```python
from build123d import *

# Parameters (mm, degrees)
CROQUIS3_R            = 2.25
CROQUIS3_R_2          = 1.25
CORTAR_EXTRUIR1_DEPTH = 2.5
CORTAR_EXTRUIR2_DEPTH = 8


with BuildPart() as part:
    # Croquis2 → Revolución1 (revolve)
    with BuildSketch(Plane.XY):
        Polygon((0, 0), (1, 0), (1, 2.05), (6.75, 2.05), (6.75, 6.05), (1, 6.05), (1, 8.1), (12.4, 8.1), (12.4, 61.6), (3.5, 61.6), (3.5, 64.2), (2, 64.2), (2, 73.7), (0, 73.7), align=None)
    revolve(axis=Axis((0, 73.7, 0), (0, -1, 0)))

    # Croquis3 → Cortar-Extruir1 (cut)
    with BuildSketch(Plane(origin=(0, 61.6, 0), x_dir=(1, 0, 0), z_dir=(0, 1, 0))):
        with Locations((8.75, 0)):
            Circle(CROQUIS3_R)
        with Locations((-8.75, 0)):
            Circle(CROQUIS3_R)
        with Locations((0, 8.5)):
            Circle(CROQUIS3_R_2)
        with Locations((0, -8.5)):
            Circle(CROQUIS3_R_2)
    extrude(amount=-CORTAR_EXTRUIR1_DEPTH, mode=Mode.SUBTRACT)

    # Croquis4 → Cortar-Extruir2 (cut)
    with BuildSketch(Plane(origin=(0, 73.7, 0), x_dir=(1, 0, 0), z_dir=(0, 1, 0))):
        Polygon((1.5, 50.388324137), (1.5, 1.322875656), (1.5, -1.322875656), (1.5, -50.388324137), (99.630896962, -50.388324137), (99.630896962, 50.388324137), align=None)
    extrude(amount=-CORTAR_EXTRUIR2_DEPTH, mode=Mode.SUBTRACT)


solid = part.part
```
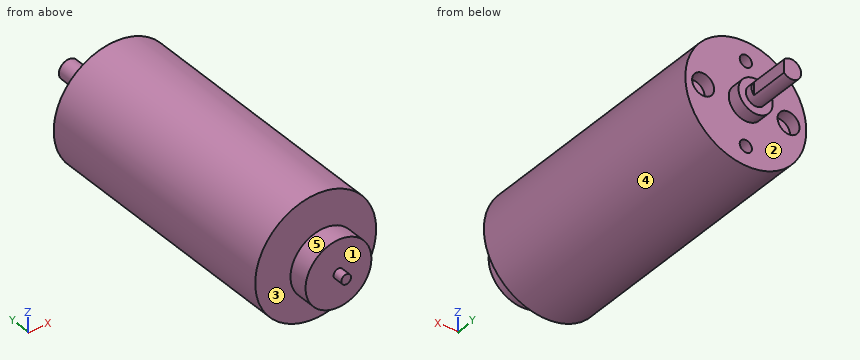
CAD build for the part. Positions are in the model's coordinates, mm. Face numbers are marked on the shaded views. A direction names the side the tool comes from. Round coordinates to 2 decimals unless told otherwise and drop trailing zeros. Order: outer loops, then holes, each group sorted by start corner. A loop starts at its lowest first (then second) coordinate and runs counter-clockwise, first axis right, second up.
Q1. Slice it at D-D (y = 39.5). Write the cut outline in (x, z), and give its area (3 significant figures).
Q2. Slice it at B-B (x = -10). Write the cut outline in (y, z), and give its area (3 significant figures).
Q3. Drop flat-ended pins along their axis: pin 1 (8 mm diameter, centred on y = 15, z = 6, fed in from +X); pin 2 (4 mm diameter, centred on x = 8.75, z = 0, fed in from +Y); pin 3 (2 mm diameter, centred on y = 48.5, z = -6, fed in from -X). Give the stop position or say it passes through.
Q4. Wall check: L1, parallel to Z at x = 0, y = 60.75; L2, parallel to Y at x = -2, z = -4.5; L3, parallel to Y at x = 8.5, z = 0.75. Give the ranges that are in metal, low to high.
Q5. Two-plate mould, pull along Y, no slides. Class the marked faces 1, 2 and 3: pulls with the +Y half, pulls with the -Y half, needs draft (parallel to the pull), parting line crosses it, or undercut.
Q6. Slice it at C-C (x = 5.75). Write the cut outline in (y, z).
Q7. Which spindle directions (+Z, -Z, +X, -X, +Y, -Y) get a long thin tool onto all of the face, cutting with end or side? Do the marked faces 4 and 5. Say none if no direction does.
Results below:
1. outline: circle Ø24.8 at (0, 0)
1. area: 483 mm2
2. outline: (8.1, -7.33) - (61.6, -7.33) - (61.6, -1.87) - (59.1, -1.87) - (59.1, 1.87) - (61.6, 1.87) - (61.6, 7.33) - (8.1, 7.33) - close
2. area: 775 mm2
3. pin 1: stops at x = 12.24
3. pin 2: stops at y = 59.1
3. pin 3: stops at x = -11.35
4. L1: z = -12.4 to -9.75, -7.25 to 7.25, 9.75 to 12.4
4. L2: y = 2.05 to 6.05, 8.1 to 61.6
4. L3: y = 8.1 to 59.1
5. face 1: pulls with the -Y half
5. face 2: pulls with the +Y half
5. face 3: undercut
6. outline: (2.05, -3.54) - (6.05, -3.54) - (6.05, 3.54) - (2.05, 3.54) - close; (8.1, -10.99) - (61.6, -10.99) - (61.6, 10.99) - (8.1, 10.99) - close
7. face 4: +Y, -Y
7. face 5: -Y
